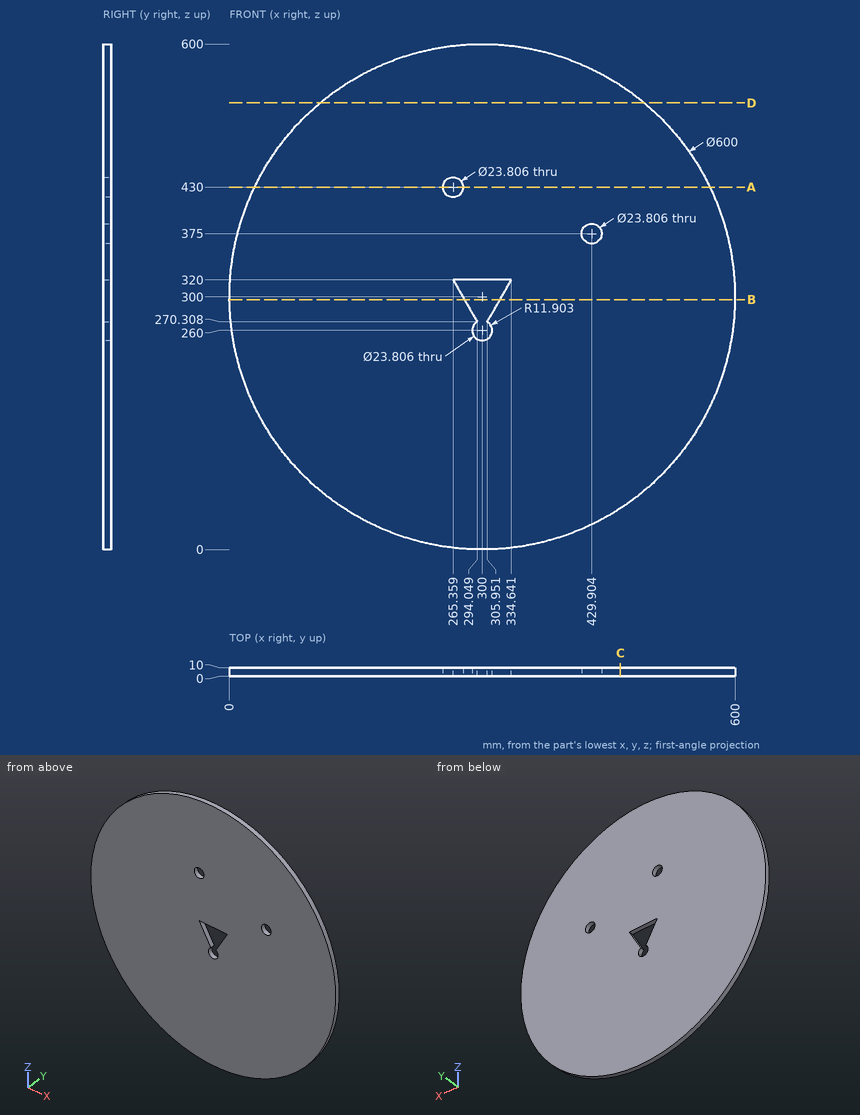
Geometry: see drawing. Coordinates: mm, zero at the bounding-box minimum. Round coordinates to 2 decimals unless told otherwise and drop trailing zeros. Order: outer loops, then holes, each group sorted by start corner. A loop starts at its lowest first (then second) coordinate and runs counter-clockwise, first axis right, second up. Notation, with made-up numbers: (36.25, 21.5) -> (86.25, 21.5) arc R17 ccw to (86.25, 50.5) -> close; hole circle Ø8 at (27.25, 79.25). An arc over 180 degrees is marked (long way). Write each question's results on one line, items separated by ' | '.
Q1. Section query D-D (z = 530). Output: boundary loops of the cut face in (x, y), and give its area (3 significant figures).
Response values:
outline: (107.39, 0) -> (492.61, 0) -> (492.61, 10) -> (107.39, 10) -> close | area: 3,850 mm²
Q2. Ray query, line 1 along Z through (x, y) = (435, 3.25) (1 decimal); line 2 along X through (y, z) = (6.5, 260); line 3 along X through (y, z) = (2.75, 430) (1 decimal). Return the intervals inside material, ascending.
Response values:
line 1: 32.1 to 364.2, 385.8 to 567.9 | line 2: 2.68 to 288.1, 311.9 to 597.32 | line 3: 29.6 to 253.5, 277.3 to 570.4
Q3. Pin query (flat end, axial travel): pin 1 Ø1 at (y, z) = (8.5, 86) entering from +X (1 decimal); pin 2 Ø3 at (y, z) = (5.5, 370) entering from -X (1 decimal); pin 3 Ø6 at (x, y) = (320, 6) entering from +Z; pin 4 Ø1.5 at (x, z) = (366.5, 460.5) entering from -Y. Return the tip coordinate at first contact, or that it passes through.
Response values:
pin 1: x = 510.8 | pin 2: x = 7.9 | pin 3: z = 599.52 | pin 4: y = 0
Q4. Section query C-C (x = 464). Output: boundary loops of the cut face in (y, z) (1 decimal).
Response values:
outline: (0, 48.8) -> (10, 48.8) -> (10, 551.2) -> (0, 551.2) -> close
Q5. Section query A-A (z = 430). Output: boundary loops of the cut face in (x, y), and give its area (3 significant figures).
Response values:
outline: (29.63, 0) -> (253.46, 0) -> (253.46, 10) -> (29.63, 10) -> close; (277.26, 0) -> (570.37, 0) -> (570.37, 10) -> (277.26, 10) -> close | area: 5,170 mm²
Q6. Section query B-B (z = 296.5). Output: boundary loops of the cut face in (x, y).
Response values:
outline: (0.02, 0) -> (278.93, 0) -> (278.93, 10) -> (0.02, 10) -> close; (321.07, 0) -> (599.98, 0) -> (599.98, 10) -> (321.07, 10) -> close
